from build123d import *

# Parameters (mm, degrees)
BOSS_EXTRUDE1_DEPTH = 8
BOSS_EXTRUDE2_DEPTH = 6
SKETCH2_R           = 3
CUT_EXTRUDE2_DEPTH  = 12


with BuildPart() as part:
    # Sketch1 → Boss-Extrude1 (new, symmetric)
    with BuildSketch(Plane(origin=(0, 0, 0), x_dir=(1, 0, 0), z_dir=(0, 1, 0))):
        with BuildLine():
            ThreePointArc((10.062305899, 3), (-1.018831921, 10.450453651), (-10.45227248, 1))
            Line((-10.45227248, 1), (-30.5, 1))
            Line((-30.5, 1), (-30.5, 5))
            Line((-30.5, 5), (-14.142135624, 5))
            ThreePointArc((-14.142135624, 5), (15, 0), (-14.142135624, -5))
            Line((-14.142135624, -5), (-30.5, -5))
            Line((-30.5, -5), (-30.5, -1))
            Line((-30.5, -1), (-10.45227248, -1))
            ThreePointArc((-10.45227248, -1), (-1.018831921, -10.450453651), (10.062305899, -3))
            Line((10.062305899, -3), (13.5, -3))
            Line((13.5, -3), (13.5, 3))
            Line((13.5, 3), (10.062305899, 3))
        make_face()
    extrude(amount=BOSS_EXTRUDE1_DEPTH, both=True)

    # Sketch1_4 → Boss-Extrude2 (add, symmetric)
    with BuildSketch(Plane(origin=(0, 0, 0), x_dir=(1, 0, 0), z_dir=(0, 1, 0))):
        with BuildLine():
            ThreePointArc((54.434579439, -9.956232283), (63.5, 0), (54.434579439, 9.956232283))
            Line((54.434579439, 9.956232283), (1.401869159, 14.934348424))
            ThreePointArc((1.401869159, 14.934348424), (15, 0), (1.401869159, -14.934348424))
            Line((1.401869159, -14.934348424), (54.434579439, -9.956232283))
        make_face()
    extrude(amount=BOSS_EXTRUDE2_DEPTH, both=True)

    # Sketch2 → Cut-Extrude2 (cut)
    with BuildSketch(Plane.XY.offset(5)):
        with Locations((-22.5, 0)):
            Circle(SKETCH2_R)
        with BuildLine():
            Line((-22.5, 8), (-22.5, 10.643526933))
            Line((-22.5, 10.643526933), (-32.266859183, 10.643526933))
            Line((-32.266859183, 10.643526933), (-32.266859183, -8))
            Line((-32.266859183, -8), (-32.266859183, -9.04856402))
            Line((-32.266859183, -9.04856402), (-22.5, -9.04856402))
            Line((-22.5, -9.04856402), (-22.5, -8))
            ThreePointArc((-22.5, -8), (-30.5, 0), (-22.5, 8))
        make_face()
    extrude(amount=-CUT_EXTRUDE2_DEPTH, mode=Mode.SUBTRACT)

    # Sketch4 → Cut-Loft1 section 0
    with BuildSketch(Plane.XZ.offset(6)):
        with BuildLine():
            Line((38.5, -5), (48.5, -5))
            Line((48.5, -5), (48.5, 5))
            Line((48.5, 5), (38.5, 5))
            Line((38.5, 5), (38.5, -5))
        make_face()
    # Sketch3 → Cut-Loft1 section 1
    with BuildSketch(Plane(origin=(0, 6, 0), x_dir=(1, 0, 0), z_dir=(0, 1, 0))):
        with BuildLine():
            Line((39.5, -4), (47.5, -4))
            Line((47.5, -4), (47.5, 4))
            Line((47.5, 4), (39.5, 4))
            Line((39.5, 4), (39.5, -4))
        make_face()
    loft(mode=Mode.SUBTRACT)


solid = part.part
For this review, take the finished solid that the model builds, in its own axes (mm). A direction names the side the tool comes from. Coordinates: 2 decimals unless noted, no trailing zeros. Loops run counter-clockwise (first coordinate to the right, second up) from the corner with the lowest first, then second, coordinate; pieces in that order, holes last. Notation, with made-up numbers: (-0.5, -5) - (4.5, -5) arc R17 ccw to (4.5, 8) - close; hole circle Ø3 at (1.5, 42.5). An arc over 180 degrees is marked (long way). Return JSON: item names as keys, results as strings.
Item 1: Insertion check: pin 1 (2 mm diameter, centred on x = 41.5, y = -5, fed in from -Z); pin 2 (10 mm diameter, centred on x = 49, z = -7.5, fed in from -Y); pin 3 (5 mm diameter, centred on x = -18, y = 3, fed in from +Z). Each pin has a flat end and moves straight along its axis. Give the tip position at first contact, or say it passes through.
Determined:
{"pin 1": "stops at z = -11.26", "pin 2": "stops at y = -6", "pin 3": "stops at z = 5"}
Item 2: Take a section at C-C (y = 0). State how many separate pieces and enclosed holes the cut face has, then the cut area to 3 significant figures.
Determined:
{"separate pieces": "3", "enclosed holes": "1", "area": "1,480 mm2"}
Item 3: Take a section at B-B (z = -7). Give the boundary of the cut face in (x, y), then the cut area to 3 significant figures.
Determined:
{"outline": "(-13.27, -8) - (-7.83, -8) - (-7.83, 8) - (-13.27, 8) - close; (7.83, -8) - (13.27, -8) - (13.27, -6) - (60.64, -6) - (60.64, 6) - (13.27, 6) - (13.27, 8) - (7.83, 8) - close", "area": "743 mm2"}
Item 4: For faces 1 (the flat face through (12, 0, -3)), 2 (the flat face through (-19, 0, -5)), 3 (the flat face through (-19, 0, 5)), 4 (the cylindrical face through (-25.5, 0.1, -3)), 5 (the flat face through (-18, 0, -1)), list the 3-axis set-ups (+Z, -Z, +X, -X, +Y, -Y) from which the entire face can be reached by the end or side of a thin tool; tool diameter is ignored.
Determined:
{"face 1": "+Y, -Y", "face 2": "-Z, -X, +Y, -Y", "face 3": "+Z, -X, +Y, -Y", "face 4": "+Z, -Z", "face 5": "-X, +Y, -Y"}
Item 5: Mouldability with a two-part tool opening along Z and no side actions: class faces 6 (the cylindrical face through (-30.498, -0.176, -2.972)), 7 (the flat face through (-18, 0, 1)), 8 (the flat face through (27.55, 0.08, 12.48)) as pulls with the +Z half, pulls with the -Z half, needs draft (parallel to the pull), parting line crosses it, or undercut.
Determined:
{"face 6": "needs draft", "face 7": "undercut", "face 8": "pulls with the +Z half"}
Item 6: Take a section at D-D (x = 11.5). Give the boundary of the cut face in (y, z).
Determined:
{"outline": "(-8, -9.63) - (-6, -9.63) - (-6, -13.99) - (6, -13.99) - (6, -9.63) - (8, -9.63) - (8, -3) - (-8, -3) - close; (-8, 3) - (8, 3) - (8, 9.63) - (6, 9.63) - (6, 13.99) - (-6, 13.99) - (-6, 9.63) - (-8, 9.63) - close"}
Item 7: Take a section at A-A (x = 0). Give the boundary of the cut face in (y, z).
Determined:
{"outline": "(-8, -15) - (8, -15) - (8, -10.5) - (-8, -10.5) - close; (-8, 10.5) - (8, 10.5) - (8, 15) - (-8, 15) - close"}
Item 8: For line 1 (Y direction, x = -22.5, z = 3.95); line 2 (Z direction, x = -15, y = -6.75); line 3 (X direction, y = 0.5, z = 4.5), list the stretches that pass through material, from the lowest coordinate up.
Determined:
{"line 1": "y = -8 to -3, 3 to 8", "line 2": "z = -5 to -1, 1 to 5", "line 3": "x = -30.48 to -25.46, -19.54 to -9.49, 9.49 to 62.43"}
